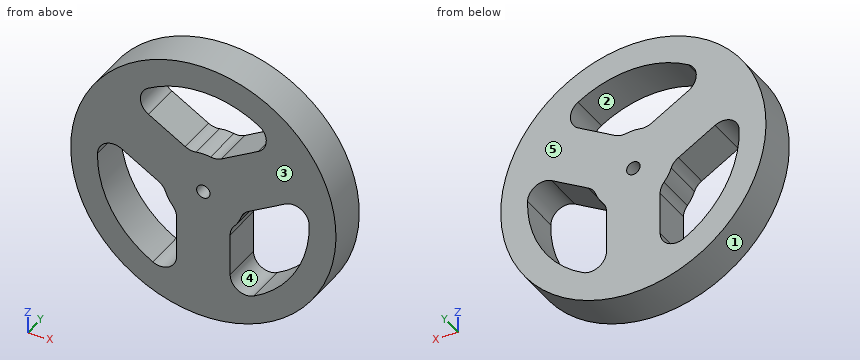
from build123d import *

# Parameters (mm, degrees)
SZKIC1_R                    = 49.5
SZKIC1_R_2                  = 39.5
SZKIC1_R_3                  = 15
SZKIC1_R_4                  = 2.5
DODANIE_WYCI_GNI_CIE1_DEPTH = 15
ZAOKR_GLENIE1_R             = 6


with BuildPart() as part:
    # Szkic1 → Dodanie-wyciągnięcie1 (new body)
    # profile 1 of 6: a face of its own
    with BuildSketch(Plane(origin=(0, 0, 0), x_dir=(1, 0, 0), z_dir=(0, 1, 0))):
        with Locations(Location((0, 0, 0), (0, 0, 270))):
            Circle(SZKIC1_R)
        Circle(SZKIC1_R_2, mode=Mode.SUBTRACT)
    # profile 2 of 6: a face of its own
    with BuildSketch(Plane(origin=(0, 0, 0), x_dir=(1, 0, 0), z_dir=(0, 1, 0))):
        with BuildLine():
            ThreePointArc((-10, 11.180339887), (-5.352331347, 14.012585384), (0, 15))
            Line((0, 15), (0, 39.5))
            ThreePointArc((0, 39.5), (-5.041225271, 39.176983648), (-10, 38.213217609))
            Line((-10, 38.213217609), (-10, 11.180339887))
        make_face()
    # profile 3 of 6: a face of its own
    with BuildSketch(Plane(origin=(0, 0, 0), x_dir=(1, 0, 0), z_dir=(0, 1, 0))):
        with BuildLine():
            Line((0, 39.5), (0, 15))
            ThreePointArc((0, 15), (5.352331347, 14.012585384), (10, 11.180339887))
            Line((10, 11.180339887), (10, 38.213217609))
            ThreePointArc((10, 38.213217609), (5.041225271, 39.176983648), (0, 39.5))
        make_face()
    # profile 4 of 6: a face of its own
    with BuildSketch(Plane(origin=(0, 0, 0), x_dir=(1, 0, 0), z_dir=(0, 1, 0))):
        with BuildLine():
            Line((38.093617209, -10.446354766), (14.682458366, 3.070084094))
            ThreePointArc((14.682458366, 3.070084094), (14.920403404, 1.54323111), (15, 0))
            ThreePointArc((15, 0), (12.149832828, -8.796679047), (4.682458366, -14.250423982))
            Line((4.682458366, -14.250423982), (28.093617209, -27.766862842))
            ThreePointArc((28.093617209, -27.766862842), (34.208003449, -19.75), (38.093617209, -10.446354766))
        make_face()
    # profile 5 of 6: a face of its own
    with BuildSketch(Plane(origin=(0, 0, 0), x_dir=(1, 0, 0), z_dir=(0, 1, 0))):
        Circle(SZKIC1_R_3)
        with Locations(Location((0, 0, 0), (0, 0, 270))):
            Circle(SZKIC1_R_4, mode=Mode.SUBTRACT)
    # profile 6 of 6: a face of its own
    with BuildSketch(Plane(origin=(0, 0, 0), x_dir=(1, 0, 0), z_dir=(0, 1, 0))):
        with BuildLine():
            ThreePointArc((-4.682458366, -14.250423982), (-12.990381057, -7.5), (-14.682458366, 3.070084094))
            Line((-14.682458366, 3.070084094), (-38.093617209, -10.446354766))
            ThreePointArc((-38.093617209, -10.446354766), (-34.208003449, -19.75), (-28.093617209, -27.766862842))
            Line((-28.093617209, -27.766862842), (-4.682458366, -14.250423982))
        make_face()
    extrude(amount=DODANIE_WYCI_GNI_CIE1_DEPTH)

    # Zaokrąglenie1
    zaokr_glenie1_edges = [part.edges().sort_by_distance(p)[0] for p in [
        (14.682458366, 7.5, -3.070084094),
        (38.093617209, 7.5, 10.446354766),
        (10, 7.5, -38.213217609),
        (10, 7.5, -11.180339887),
        (-10, 7.5, -38.213217609),
        (-38.093617209, 7.5, 10.446354766),
        (-14.682458366, 7.5, -3.070084094),
        (-10, 7.5, -11.180339887),
        (-28.093617209, 7.5, 27.766862842),
        (28.093617209, 7.5, 27.766862842),
        (4.682458366, 7.5, 14.250423982),
        (-4.682458366, 7.5, 14.250423982),
    ]]
    fillet(zaokr_glenie1_edges, radius=ZAOKR_GLENIE1_R)


solid = part.part
Can you work these out from the model? Positions are in its coordinate system, mm. Face numbers are marked on the shaded views. A direction names the side the tool comes from. Round coordinates to 2 decimals unless told otherwise and drop trailing zeros. Loops run counter-clockwise (first coordinate to the right, second up) from the corner with the lowest first, then second, coordinate; pieces in that order, holes last. Notation, with made-up numbers: (9.5, -1) - (41.5, -1) arc R19 ccw to (41.5, 11) - close; hole circle Ø1 at (56.5, 49.25). An arc over 180 degrees is marked (long way). Use CSV: the item, a comma, the result in double quotes. Start each with the question number.
1) We'd pull the mould along X, two halves only. Please class the marked faces 1, 2 and 3: released by +X, released by -X, zero draft, split by the parting line, or undercut.
2) If we section it at A-A on y = 10.25: Write out the boundary of the cut face in (x, z).
3) If we section it at C-C on x = 28.5: Write out the boundary of the cut face in (y, z), plus the area to 3 significant figures.
4) For the marked faces 4 and 5, which set-ups out of +Z, -Z, +X, -X, +Y, -Y let a thin tool reach every point of the face, with its end or its side?
5) Please list where these lines run through material, in increasing order: probe 1 along X at (y, z) = (13.5, -19.5); probe 2 along X at (y, z) = (13, -5.5); probe 3 along X at (y, z) = (5.5, 0). Write a range as [from, to].
6) If we section it at D-D on z = 21: Write out the boundary of the cut face in (x, y), plus the area to 3 significant figures.
7) If we section it at B-B on x = 0: Write out the boundary of the cut face in (y, z).
8) For pin 1 Ø4.5 at (y, z) = (9, -23.5) entering from +X; pin 2 Ø6 at (y, z) = (6.5, -32) entering from +X; pin 3 Ø6 at (y, z) = (7.5, 0.5) entering from -X; pin 4 Ø8 at (x, z) = (0, 0) entering from -Y, each with a flat end and sliding along its axis, tell me the tip position at first contact or that it passes through.
Geometry results:
1,face 1,"split by the parting line"
1,face 2,"undercut"
1,face 3,"zero draft"
2,outline,"circle Ø99 at (0, 0); hole (-39.49, 1.01) arc R39.5 ccw to (-18.87, -34.7) arc R6 ccw to (-10, -29.43) - (-10, -13.6) arc R6 ccw to (-11.43, -9.72) arc R15 cw to (-14.13, -5.04) arc R6 ccw to (-16.78, -1.86) - (-30.49, 6.06) arc R6 ccw to start; hole (-20.62, 33.69) arc R6 ccw to (-20.49, 23.38) - (-6.78, 15.46) arc R6 ccw to (-2.7, 14.76) arc R15 cw to (2.7, 14.76) arc R6 ccw to (6.78, 15.46) - (20.49, 23.38) arc R6 ccw to (20.62, 33.69) arc R39.5 ccw to start; hole circle Ø5 at (0, 0); hole (10, -29.43) arc R6 ccw to (18.87, -34.7) arc R39.5 ccw to (39.49, 1.01) arc R6 ccw to (30.49, 6.06) - (16.78, -1.86) arc R6 ccw to (14.13, -5.04) arc R15 cw to (11.43, -9.72) arc R6 ccw to (10, -13.6) - close"
3,outline,"(0, -40.47) - (15, -40.47) - (15, -27.35) - (0, -27.35) - close; (0, 4.91) - (15, 4.91) - (15, 40.47) - (0, 40.47) - close"
3,area,"730 mm2"
4,face 4,"+Y, -Y"
4,face 5,"+Z, -Z, +X, -X, +Y"
5,probe 1,"x = [-45.5, -34.35], [-10, 10], [34.35, 45.5]"
5,probe 2,"x = [-49.19, -39.12], [-13.96, 13.96], [39.12, 49.19]"
5,probe 3,"x = [-49.5, -39.5], [-20, -2.5], [2.5, 20], [39.5, 49.5]"
6,outline,"(-44.82, 0) - (-16.37, 0) - (-16.37, 15) - (-44.82, 15) - close; (16.37, 0) - (44.82, 0) - (44.82, 15) - (16.37, 15) - close"
6,area,"854 mm2"
7,outline,"(0, -49.5) - (15, -49.5) - (15, -2.5) - (0, -2.5) - close; (0, 2.5) - (15, 2.5) - (15, 15) - (0, 15) - close; (0, 39.5) - (15, 39.5) - (15, 49.5) - (0, 49.5) - close"
8,pin 1,"stops at x = 44.71"
8,pin 2,"stops at x = 40.12"
8,pin 3,"stops at x = -49.5"
8,pin 4,"stops at y = 0"
